Part model, mm, in its own coordinate system. Face numbers are marked on the shaded views. Coordinates: 2 decimals unless noted, no trailing zeros.
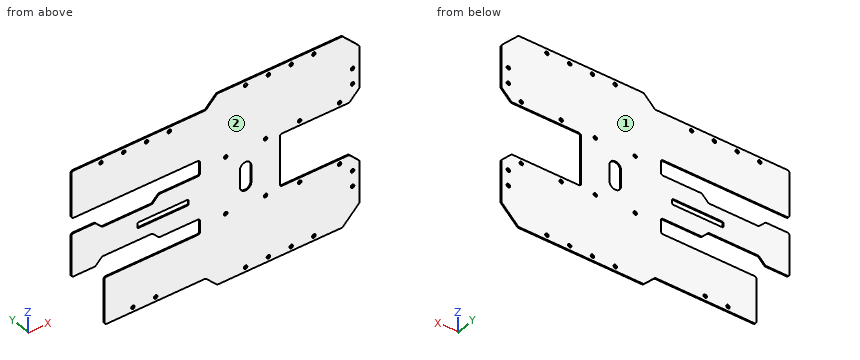
from build123d import *
from build123d.topology import SkipClean

# Parameters (mm, degrees)
SKETCH_1_W          = 70
SKETCH_1_H          = 70
SKETCH_1_R          = 1.6
EXTRUDE_1_DEPTH     = 1
EXTRUDE_2_DEPTH     = 1
SKETCH_5_W          = 113
SKETCH_5_H          = 30
EXTRUDE_5_DEPTH     = 1
SKETCH_6_R          = 1.55
CUT_EXTRUDE_1_DEPTH = 1
SKETCH_7_W          = 15
SKETCH_7_H          = 17.5
EXTRUDE_6_DEPTH     = 1
SKETCH_8_W          = 40
SKETCH_8_H          = 4
SKETCH_8_W_2        = 12
SKETCH_8_W_3        = 27
EXTRUDE_7_DEPTH     = 1
CHAMFER_1_SIZE      = 4
SKETCH_9_W          = 15
SKETCH_9_H          = 13.5
CUT_EXTRUDE_2_DEPTH = 1
CHAMFER_2_SIZE      = 6
SKETCH_10_W         = 45
SKETCH_10_H         = 5
SKETCH_10_W_2       = 70
SKETCH_10_H_2       = 46
CUT_EXTRUDE_3_DEPTH = 10
FILLET_1_R          = 1
SKETCH_11_R         = 1.55
CUT_EXTRUDE_4_DEPTH = 10
CHAMFER_3_SIZE      = 9
FILLET_2_R          = 2
SKETCH_12_R         = 1.55
CUT_EXTRUDE_5_DEPTH = 5
CUT_EXTRUDE_6_DEPTH = 10


# Some blends are built 0.0001 mm under size
with BuildPart() as part:
    # 草图1 → 凸台-拉伸1 (new body)
    with BuildSketch(Plane(origin=(0, 0, 0), x_dir=(1, 0, 0), z_dir=(0, 1, 0))):
        Rectangle(SKETCH_1_W, SKETCH_1_H)
        with Locations(Location((13, -13, 0), (0, 0, 270))):
            Circle(SKETCH_1_R, mode=Mode.SUBTRACT)
        with Locations(Location((13, 13, 0), (0, 0, 270))):
            Circle(SKETCH_1_R, mode=Mode.SUBTRACT)
        with Locations(Location((-13, 13, 0), (0, 0, 270))):
            Circle(SKETCH_1_R, mode=Mode.SUBTRACT)
        with Locations(Location((-13, -13, 0), (0, 0, 270))):
            Circle(SKETCH_1_R, mode=Mode.SUBTRACT)
    extrude(amount=EXTRUDE_1_DEPTH)

    # 草图2 → 凸台-拉伸2 (add)
    with BuildSketch(Plane.XZ):
        Polygon((35, -35), (35, -69), (20, -84), (-90, -84), (-100, -74), (-189, -74), (-189, -32.5), (-105, -32.5), (-105, 32.5), (-218, 32.5), (-218, 74), (-100, 74), (-90, 84), (20, 84), (35, 69), (35, 35), (-35, 35), (-35, -35), align=None)
    extrude(amount=-EXTRUDE_2_DEPTH)

    # 草图5 → 凸台-拉伸5 (add)
    with BuildSketch(Plane(origin=(0, 1, 0), x_dir=(1, 0, 0), z_dir=(0, 1, 0))):
        with Locations((-161.5, 0)):
            Rectangle(SKETCH_5_W, SKETCH_5_H)
    extrude(amount=-EXTRUDE_5_DEPTH)

    # 草图6 → 切除-拉伸1 (cut)
    with BuildSketch(Plane.XZ):
        with Locations(Location((-5, -80, 0), (0, 0, 270))):
            Circle(SKETCH_6_R)
        with Locations(Location((-25, -80, 0), (0, 0, 270))):
            Circle(SKETCH_6_R)
        with Locations(Location((-65, -80, 0), (0, 0, 270))):
            Circle(SKETCH_6_R)
        with Locations(Location((-45, -80, 0), (0, 0, 270))):
            Circle(SKETCH_6_R)
        with Locations(Location((-45, 80, 0), (0, 0, 90))):
            Circle(SKETCH_6_R)
        with Locations(Location((-65, 80, 0), (0, 0, 90))):
            Circle(SKETCH_6_R)
        with Locations(Location((-25, 80, 0), (0, 0, 90))):
            Circle(SKETCH_6_R)
        with Locations(Location((-5, 80, 0), (0, 0, 90))):
            Circle(SKETCH_6_R)
        with Locations(Location((-164, -70, 0), (0, 0, 270))):
            Circle(SKETCH_6_R)
        with Locations(Location((-192, 70, 0), (0, 0, 270))):
            Circle(SKETCH_6_R)
        with Locations(Location((-172, 70, 0), (0, 0, 270))):
            Circle(SKETCH_6_R)
        with Locations(Location((-152, 70, 0), (0, 0, 270))):
            Circle(SKETCH_6_R)
        with Locations(Location((-132, 70, 0), (0, 0, 270))):
            Circle(SKETCH_6_R)
        with Locations(Location((-144, -70, 0), (0, 0, 270))):
            Circle(SKETCH_6_R)
    extrude(amount=-CUT_EXTRUDE_1_DEPTH, mode=Mode.SUBTRACT)

    # 草图7 → 凸台-拉伸6 (add)
    with BuildSketch(Plane.XZ):
        with Locations((-210.5, 23.75)):
            Rectangle(SKETCH_7_W, SKETCH_7_H)
    extrude(amount=-EXTRUDE_6_DEPTH)

    # 草图8 → 凸台-拉伸7 (add)
    with BuildSketch(Plane(origin=(0, 1, 0), x_dir=(1, 0, 0), z_dir=(0, 1, 0))):
        with Locations((-125, 17)):
            Rectangle(SKETCH_8_W, SKETCH_8_H)
        with Locations((-125, -17)):
            Rectangle(SKETCH_8_W, SKETCH_8_H)
        with Locations((-197, -17)):
            Rectangle(SKETCH_8_W_2, SKETCH_8_H)
        with Locations((-204.5, 17)):
            Rectangle(SKETCH_8_W_3, SKETCH_8_H)
    extrude(amount=-EXTRUDE_7_DEPTH)

    # 倒角1
    chamfer_1_edges = [part.edges().sort_by_distance(p)[0] for p in [
        (-145, 0.5, -19),
        (-145, 0.5, 19),
    ]]
    chamfer(chamfer_1_edges, length=CHAMFER_1_SIZE - 0.0001)  # a hair under: the kernel refuses the full size

    # 草图9 → 切除-拉伸2 (cut)
    with SkipClean():  # the faces are left unmerged after this step: merging them gives an invalid solid
        with BuildSketch(Plane(origin=(0, 1, 0), x_dir=(1, 0, 0), z_dir=(0, 1, 0))):
            with Locations((-210.5, -25.75)):
                Rectangle(SKETCH_9_W, SKETCH_9_H)
            Polygon((-145, -15), (-147, -13), (-191, -13), (-191, -15), align=None)
            Polygon((-145, 15), (-191, 15), (-191, 13), (-147, 13), align=None)
        extrude(amount=-CUT_EXTRUDE_2_DEPTH, mode=Mode.SUBTRACT)

    # 倒角2
    # the kernel refuses this chamfer: 6 mm, written as the material it takes off along each edge
    with BuildSketch(Plane(origin=(-191, 16.430097928, -19), x_dir=(0.027495876610586775, 0, 0.9996219169112968), z_dir=(0, -1, 0))) as chamfer_2_piece_1_section:
        Polygon((CHAMFER_2_SIZE * 0.999621916911, CHAMFER_2_SIZE * 0.0274958766106), (-CHAMFER_2_SIZE * 0.0274958766106, CHAMFER_2_SIZE * 0.999621916911), (0, 0), align=None)
    chamfer_2_piece_1 = extrude(amount=31.860195856, mode=Mode.PRIVATE)
    chamfer_2_piece_1 = split(chamfer_2_piece_1, bisect_by=Plane(origin=(-192.982424926, 0.5, -13), z_dir=(0, 0, -1)), keep=Keep.TOP, mode=Mode.PRIVATE)
    add(chamfer_2_piece_1, mode=Mode.SUBTRACT)
    with BuildSketch(Plane(origin=(-191, 16.430097928, 19), x_dir=(-0.9996219169112968, 0, 0.02749587661058619), z_dir=(0, -1, 0))) as chamfer_2_piece_2_section:
        Polygon((CHAMFER_2_SIZE * 0.999621916911, CHAMFER_2_SIZE * 0.0274958766106), (-CHAMFER_2_SIZE * 0.0274958766106, CHAMFER_2_SIZE * 0.999621916911), (0, 0), align=None)
    chamfer_2_piece_2 = extrude(amount=31.860195856, mode=Mode.PRIVATE)
    chamfer_2_piece_2 = split(chamfer_2_piece_2, bisect_by=Plane(origin=(-192.982424926, 0.5, 13), z_dir=(0, 0, 1)), keep=Keep.TOP, mode=Mode.PRIVATE)
    add(chamfer_2_piece_2, mode=Mode.SUBTRACT)

    # 草图10 → 切除-拉伸3 (cut)
    with SkipClean():  # the faces are left unmerged after this step: merging them gives an invalid solid
        with BuildSketch(Plane(origin=(0, 1, 0), x_dir=(1, 0, 0), z_dir=(0, 1, 0))):
            with Locations((-137.5, 0)):
                Rectangle(SKETCH_10_W, SKETCH_10_H)
            Rectangle(SKETCH_10_W_2, SKETCH_10_H_2)
        extrude(amount=-CUT_EXTRUDE_3_DEPTH, mode=Mode.SUBTRACT)

    # 圆角1
    fillet_1_edges = [part.edges().sort_by_distance(p)[0] for p in [
        (-115, 0.5, -2.5),
        (-115, 0.5, 2.5),
        (-160, 0.5, 2.5),
        (-160, 0.5, -2.5),
    ]]
    fillet(fillet_1_edges, radius=FILLET_1_R)

    # 草图11 → 切除-拉伸4 (cut)
    with SkipClean():  # the faces are left unmerged after this step: merging them gives an invalid solid
        with BuildSketch(Plane.XZ):
            with Locations(Location((17.5, -27, 0), (0, 0, 270))):
                Circle(SKETCH_11_R)
            with Locations(Location((17.5, 27, 0), (0, 0, 270))):
                Circle(SKETCH_11_R)
            with Locations(Location((-17.5, 27, 0), (0, 0, 270))):
                Circle(SKETCH_11_R)
            with Locations(Location((-17.5, -27, 0), (0, 0, 270))):
                Circle(SKETCH_11_R)
            with Locations(Location((-47.5, 25, 0), (0, 0, 270))):
                Circle(SKETCH_11_R)
            with Locations(Location((-47.5, -25, 0), (0, 0, 270))):
                Circle(SKETCH_11_R)
            with Locations(Location((-82.5, -25, 0), (0, 0, 270))):
                Circle(SKETCH_11_R)
            with Locations(Location((-82.5, 25, 0), (0, 0, 270))):
                Circle(SKETCH_11_R)
        extrude(amount=-CUT_EXTRUDE_4_DEPTH, mode=Mode.SUBTRACT)

    # 倒角3
    chamfer_3_edges = [part.edges().sort_by_distance(p)[0] for p in [
        (35, 0.5, -23),
        (35, 0.5, 23),
    ]]
    chamfer(chamfer_3_edges, length=CHAMFER_3_SIZE)

    # 圆角2
    fillet_2_edges = [part.edges().sort_by_distance(p)[0] for p in [
        (-105, 0.5, -19),
        (-105, 0.5, 19),
        (-218, 0.5, -19),
        (-141.0001, 0.5, -19),
        (-141.0001, 0.5, 19),
        (-218, 0.5, 32.5),
        (-218, 0.5, 19),
        (-191, 0.5, 13),
        (-147, 0.5, 13),
        (-147, 0.5, -13),
        (-191, 0.5, -13),
        (-197, 0.5, -19),
        (-197, 0.5, 19),
        (35, 0.5, -69),
        (20, 0.5, -84),
        (-90, 0.5, -84),
        (-100, 0.5, -74),
        (-189, 0.5, -74),
        (-35, 0.5, 23),
        (-35, 0.5, -23),
        (-189, 0.5, -32.5),
        (-105, 0.5, -32.5),
        (-105, 0.5, 32.5),
        (-218, 0.5, 74),
        (-100, 0.5, 74),
        (-90, 0.5, 84),
        (20, 0.5, 84),
        (35, 0.5, 69),
        (35, 0.5, 32),
        (26, 0.5, 23),
        (35, 0.5, -32),
        (26, 0.5, -23),
    ]]
    fillet(fillet_2_edges, radius=FILLET_2_R)

    # 草图12 → 切除-拉伸5 (cut)
    with SkipClean():  # the faces are left unmerged after this step: merging them gives an invalid solid
        with BuildSketch(Plane.XZ):
            with Locations(Location((28.9, 38.2, 0), (0, 0, 270))):
                Circle(SKETCH_12_R)
            with Locations(Location((28.9, 51.8, 0), (0, 0, 270))):
                Circle(SKETCH_12_R)
            with Locations(Location((28.9, -38.2, 0), (0, 0, 270))):
                Circle(SKETCH_12_R)
            with Locations(Location((28.9, -51.8, 0), (0, 0, 270))):
                Circle(SKETCH_12_R)
        extrude(amount=-CUT_EXTRUDE_5_DEPTH, mode=Mode.SUBTRACT)

    # 草图13 → 切除-拉伸6 (cut)
    with SkipClean():  # the faces are left unmerged after this step: merging them gives an invalid solid
        with BuildSketch(Plane.XZ):
            with BuildLine():
                Line((-60, 7.5), (-60, -7.5))
                ThreePointArc((-60, -7.5), (-65, -12.5), (-70, -7.5))
                Line((-70, -7.5), (-70, 7.5))
                ThreePointArc((-70, 7.5), (-65, 12.5), (-60, 7.5))
            make_face()
        extrude(amount=-CUT_EXTRUDE_6_DEPTH, mode=Mode.SUBTRACT)


solid = part.part
Q1. Mould opens along Y. For the marked faces 1 and 2 say: pulls with the +Y half, pulls with the -Y half, needs draft (parallel to the pull), parting line crosses it, or undercut.
Results list:
face 1: pulls with the +Y half
face 2: pulls with the -Y half
Q2. Wall check: line 1 along Z through (x, y) = (-126, 0.95); line 2 along Z through (x, y) = (-172, 0.4); line 3 along Z through (x, y) = (-15.5, 0.95). Give the ranges that are in metal, low to high.
Results list:
line 1: z = -74 to -32.5, -19 to -2.5, 2.5 to 19, 32.5 to 74
line 2: z = -74 to -32.5, -13 to 13, 32.5 to 68.45, 71.55 to 74
line 3: z = -84 to -23, 23 to 84
Q3. Cut at A-A on y = 0.3. Count the separate pieces of the cut face and the enclosed holes in it, and give its area (3 significant figures).
Results list:
separate pieces: 1
enclosed holes: 28
area: 31,000 mm2
Q4. Pin check, flat tips, straight feed: pin 1 Ø1.9 at (x, z) = (-172, 70) entering from -Y; pin 2 Ø0.5 at (x, y) = (-210, 0.5) entering from +Z; pin 3 Ø0.5 at (y, z) = (0.5, -54.5) entering from -X. Stop position of each tip, or through.
Results list:
pin 1: passes through
pin 2: stops at z = 74
pin 3: stops at x = -189
